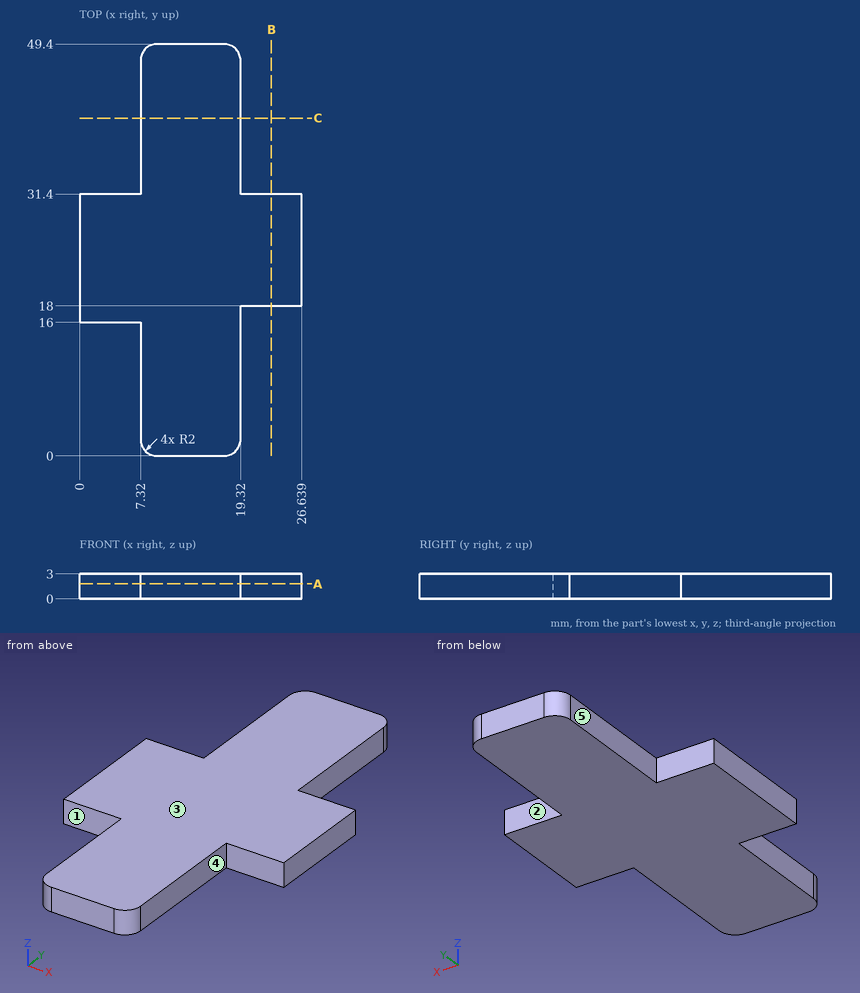
Design review of the part shown in the three views and the two pictorial views. Dimensions are in mm from the part's minimum x, y and z. A direction names the side the tool comes from. Round coordinates to 2 decimals unless told otherwise and drop trailing zeros. Loops run counter-clockwise (first coordinate to the right, second up) from the corner with the lowest first, then second, coordinate; pieces in that order, holes last. Notation, with made-up numbers: M 4.25,5.5 L 57.25,5.5 A9 ccw 57.25,18.5 Z; hole C 50.25,16.25 d5. An arc over 180 degrees is marked long. Put each result on its own line as item: value.
Q1. Consider section B-B, the plane x = 23. Give the boundary of the cut face in (y, z), then the cut area to 3 significant figures.
Result set:
outline: M 18,0 L 31.4,0 L 31.4,3 L 18,3 Z
area: 40.2 mm²
Q2. Consider section C-C, the plane y = 40.5. Give the boundary of the cut face in (x, z), then the cut area to 3 significant figures.
Result set:
outline: M 7.32,0 L 19.32,0 L 19.32,3 L 7.32,3 Z
area: 36.0 mm²
Q3. To check wall thickness, follow L1, parallel to X at y = 47.5, z = 2.35; L2, parallel to X at y = 17, z = 1.45; L3, parallel to Y at x = 5.25, z = 2.7. State the ranges of each line that lie inside material, in increasing order.
Result set:
L1: x = 7.32 to 19.32
L2: x = 0 to 19.32
L3: y = 16 to 31.4
Q4. Machinability: for the marked faces 1, 2, 3, 4 and 5, which of the approach directions +Z, -Z, +X, -X, +Y, -Y give a long, thin tool a straight path to every point of the face, cutting with its end or side? Answer none if there is none.
Result set:
face 1: +Z, -Z, -X, -Y
face 2: +Z, -Z, +X, +Y
face 3: +Z, +X, -X, +Y, -Y
face 4: +Z, -Z, +X, -Y
face 5: +Z, -Z, -X, +Y
Q5. For pin 1 (1.5 mm diameter, centred on y = 9, z = 2, fed in from -X); pin 2 (1.5 mm diameter, centred on y = 7, z = 1, fed in from +X); pin 3 (0.9 mm diameter, centred on x = 22.5, z = 1, fed in from -Y), all flat-tipped, find the tip position at first contact; note any pin that passes through.
Result set:
pin 1: stops at x = 7.32
pin 2: stops at x = 19.32
pin 3: stops at y = 18
Q6. Consider section A-A, the plane z = 1.8. Give the boundary of the cut face in (x, y).
Result set:
outline: M 0,16 L 7.32,16 L 7.32,2 A2 ccw 9.32,0 L 17.32,0 A2 ccw 19.32,2 L 19.32,18 L 26.64,18 L 26.64,31.4 L 19.32,31.4 L 19.32,47.4 A2 ccw 17.32,49.4 L 9.32,49.4 A2 ccw 7.32,47.4 L 7.32,31.4 L 0,31.4 Z
